```python
from build123d import *

# Parameters (mm, degrees)
SKETCH1_W           = 103.47926424
SKETCH1_H           = 64
BOSS_EXTRUDE1_DEPTH = 3
SKETCH2_W           = 46.52073576
SKETCH2_H           = 3
BOSS_EXTRUDE2_DEPTH = 3
FILLET1_R           = 3
SKETCH3_R           = 8.958865037
SKETCH3_R_2         = 7.958865037
EXTRUDE_THIN1_DEPTH = 2


with BuildPart() as part:
    # Sketch1 → Boss-Extrude1 (new body)
    with BuildSketch(Plane.XY):
        with Locations((11.73963212, 81.73418814)):
            Rectangle(SKETCH1_W, SKETCH1_H)
    extrude(amount=BOSS_EXTRUDE1_DEPTH)

    # Sketch2 → Boss-Extrude2 (add)
    with BuildSketch(Plane.XY.offset(3)):
        with Locations((86.73963212, 112.23418814)):
            Rectangle(SKETCH2_W, SKETCH2_H)
        with Locations((86.73963212, 51.23418814)):
            Rectangle(SKETCH2_W, SKETCH2_H)
    extrude(amount=-BOSS_EXTRUDE2_DEPTH)

    # Fillet1
    fillet1_edges = [part.edges().sort_by_distance(p)[0] for p in [
        (110, 51.23418814, 3),
        (110, 112.23418814, 3),
    ]]
    fillet(fillet1_edges, radius=FILLET1_R - 0.0001)  # a hair under: the kernel refuses the full size

    # Sketch3 → Extrude-Thin1 (add)
    with BuildSketch(Plane(origin=(23.47926424, 0, 0), x_dir=(0, 0, -1), z_dir=(1, 0, 0))):
        with Locations((-8.102432793, 81.734499249)):
            Circle(SKETCH3_R)
        with Locations((-8.102432793, 81.734499249)):
            Circle(SKETCH3_R_2, mode=Mode.SUBTRACT)
    extrude(amount=EXTRUDE_THIN1_DEPTH)


solid = part.part
```
For this review, take the finished solid that the model builds, in its own axes (mm). A direction names the side the tool comes from. Coordinates: 2 decimals unless noted, no trailing zeros. Write each loop counter-clockwise with the first axis right and the second up, starting at its lowest first coordinate (ties: lowest second). Pieces come first, ordered by that corner, then holes.
(1) Wall thickness on probe 1 along X at (y, z) = (70, 2); probe 2 along Y at (x, z) = (93.5, 1.5); probe 3 along Z at (x, y) = (6.5, 75): over which ranges is each line inside the solid? List them lowest first.
(2) The part is to be moulded in two halves that separate along Y. For faces 4 (the face through (34, 113.734, 2)), 5 (the face through (23.479, 81.8, 16.3)), 6 (the face through (24.465, 81.987, 16.057)), 7 (the face through (63.479, 81, 1)), say which applies: +Y half, -Y half, draft (parallel to the pull), parting line (faces both ways), or undercut.
(3) Add section C-C on z = 1.5. Give the boundary of the cut face in (x, y), then the cut area to 3 significant figures.
(4) Add section B-B on z = 13.5. Give the boundary of the cut face in (x, y).
(5) Add section A-A on x = 89. Give the boundary of the cut face in (y, z), then the cut area to 3 significant figures.
(6) Add section D-D on x = 50. Give the boundary of the cut face in (y, z), then the cut area to 3 significant figures.
(7) Tool access review of faces 1 (the face through (25.479, 81.8, 16.3)), 2 (the face through (86, 110.734, 2)), 3 (the face through (-40, 81, 1)): name each direction out of +Z, -Z, +X, -X, +Y, -Y from which nothing blocks a thin tool from reaching the whole face with its end or side.
(8) For pin 1 Ø0.9 at (y, z) = (82.5, -0.5) entering from +X; pin 2 Ø5 at (y, z) = (69, 13) entering from -X; pin 3 Ø3 at (x, y) = (64, 87) entering from +Z; pin 4 Ø0.7 at (y, z) = (80, -0.5) entering from -X, all flat-tipped, find the tip position at first contact; note any pin that passes through.
Answer sheet:
1. probe 1: x = -40 to 63.48
1. probe 2: y = 49.73 to 52.73, 110.73 to 113.73
1. probe 3: z = 0 to 3
2. face 4: +Y half
2. face 5: draft
2. face 6: undercut
2. face 7: undercut
3. outline: (-40, 49.73) - (109.6, 49.73) - (109.6, 52.73) - (63.48, 52.73) - (63.48, 110.73) - (109.6, 110.73) - (109.6, 113.73) - (-40, 113.73) - close
3. area: 6,900 mm2
4. outline: (23.48, 74.58) - (25.48, 74.58) - (25.48, 75.89) - (23.48, 75.89) - close; (23.48, 87.58) - (25.48, 87.58) - (25.48, 88.88) - (23.48, 88.88) - close
5. outline: (49.73, 0) - (52.73, 0) - (52.73, 3) - (49.73, 3) - close; (110.73, 0) - (113.73, 0) - (113.73, 3) - (110.73, 3) - close
5. area: 18.0 mm2
6. outline: (49.73, 0) - (113.73, 0) - (113.73, 3) - (49.73, 3) - close
6. area: 192 mm2
7. face 1: +Z, +X, +Y, -Y
7. face 2: +Z, -Z, +X
7. face 3: +Z, -Z, -X, +Y, -Y
8. pin 1: stops at x = 25.48
8. pin 2: passes through
8. pin 3: stops at z = 3
8. pin 4: stops at x = 23.48
